from build123d import *

# Parameters (mm, degrees)
SKETCH1_W           = 101.6
SKETCH1_H           = 79
BOSS_EXTRUDE1_DEPTH = 3


with BuildPart() as part:
    # Sketch1 → Boss-Extrude1 (new body)
    with BuildSketch(Plane(origin=(0, 0, 0), x_dir=(1, 0, 0), z_dir=(0, 1, 0))):
        with Locations((44.42740929, 26.5)):
            Rectangle(SKETCH1_W, SKETCH1_H)
        with BuildLine():
            Line((9.87740929, 51.5), (9.87740929, 48.5))
            ThreePointArc((9.87740929, 48.5), (6.62740929, 45.25), (3.37740929, 48.5))
            Line((3.37740929, 48.5), (3.37740929, 51.5))
            ThreePointArc((3.37740929, 51.5), (6.62740929, 54.75), (9.87740929, 51.5))
        make_face(mode=Mode.SUBTRACT)
        with BuildLine():
            Line((9.87740929, 1.5), (9.87740929, -1.5))
            ThreePointArc((9.87740929, -1.5), (6.62740929, -4.75), (3.37740929, -1.5))
            Line((3.37740929, -1.5), (3.37740929, 1.5))
            ThreePointArc((3.37740929, 1.5), (6.62740929, 4.75), (9.87740929, 1.5))
        make_face(mode=Mode.SUBTRACT)
        with BuildLine():
            Line((59.87740929, 1.5), (59.87740929, -1.5))
            ThreePointArc((59.87740929, -1.5), (56.62740929, -4.75), (53.37740929, -1.5))
            Line((53.37740929, -1.5), (53.37740929, 1.5))
            ThreePointArc((53.37740929, 1.5), (56.62740929, 4.75), (59.87740929, 1.5))
        make_face(mode=Mode.SUBTRACT)
        with BuildLine():
            Line((85.47740929, 51.5), (85.47740929, 48.5))
            ThreePointArc((85.47740929, 48.5), (82.22740929, 45.25), (78.97740929, 48.5))
            Line((78.97740929, 48.5), (78.97740929, 51.5))
            ThreePointArc((78.97740929, 51.5), (82.22740929, 54.75), (85.47740929, 51.5))
        make_face(mode=Mode.SUBTRACT)
        with BuildLine():
            Line((78.97740929, 1.5), (78.97740929, -1.5))
            ThreePointArc((78.97740929, -1.5), (82.22740929, -4.75), (85.47740929, -1.5))
            Line((85.47740929, -1.5), (85.47740929, 1.5))
            ThreePointArc((85.47740929, 1.5), (82.22740929, 4.75), (78.97740929, 1.5))
        make_face(mode=Mode.SUBTRACT)
        with BuildLine():
            Line((28.97740929, 1.5), (28.97740929, -1.5))
            ThreePointArc((28.97740929, -1.5), (32.22740929, -4.75), (35.47740929, -1.5))
            Line((35.47740929, -1.5), (35.47740929, 1.5))
            ThreePointArc((35.47740929, 1.5), (32.22740929, 4.75), (28.97740929, 1.5))
        make_face(mode=Mode.SUBTRACT)
    extrude(amount=BOSS_EXTRUDE1_DEPTH)


solid = part.part
Model file for the job. Use its own axes, mm. A direction names the side the tool comes from. Coordinates: 2 decimals unless noted, no trailing zeros. Order: outer loops, then holes, each group sorted by start corner. A loop starts at its lowest first (then second) coordinate and runs counter-clockwise, first axis right, second up. Notation, with made-up numbers: (-1, 86.25) -> (5, 86.25) arc R19 cw to (5, 121.25) -> close; hole circle Ø3 at (89, 73). An arc over 180 degrees is marked (long way). Return JSON: item names as keys, results as strings. Group by question number.
Item 1: Saw through at C-C on x = 82.5. Write the cut outline in (y, z), then the cut area to 3 significant figures.
Item 2: Saw through at A-A on y = 1.35. Write the cut outline in (x, z).
Item 3: Wall check: line 1 along X through (y, z) = (0.35, -53); line 2 along Z through (x, y) = (55, 0.35); line 3 along Z through (x, y) = (7.5, 1.1). Give the ranges that are in metal, low to high. Write a range as [from, to].
Item 4: Saw through at D-D on z = -3. Write the cut outline in (x, y).
Item 5: Tool access for faces 4 (the flat face through (59.877, 1, 0)), 5 (the flat face through (95.227, 1, -26)): list every direction of +Z, -Z, +X, -X, +Y, -Y with a clear straight run to the whole face (end or side of a thin tool).
Item 6: Saw through at B-B on z = -46.5. Write the cut outline in (x, y), then the cut area to 3 significant figures.
Item 7: Pull direction Z, two halves, no side cores. Call faces 1 (the cylindrical face through (56.7, 1.48, 4.75)), 2 (the flat face through (44, 0, -27)), 3 (the flat face through (44, 1, -66)): pulls with the +Z half, pulls with the -Z half, needs draft (parallel to the pull), parting line crosses it, or undercut.
Values found:
{
 "1": {"outline": "(0, -66) -> (3, -66) -> (3, -54.74) -> (0, -54.74) -> close; (0, -45.26) -> (3, -45.26) -> (3, -4.74) -> (0, -4.74) -> close; (0, 4.74) -> (3, 4.74) -> (3, 13) -> (0, 13) -> close", "area": "180 mm2"},
 "2": {"outline": "(-6.37, -66) -> (95.23, -66) -> (95.23, 13) -> (-6.37, 13) -> close; hole (3.38, -51.5) arc R3.25 ccw to (9.88, -51.5) -> (9.88, -48.5) arc R3.25 ccw to (3.38, -48.5) -> close; hole (3.38, -1.5) arc R3.25 ccw to (9.88, -1.5) -> (9.88, 1.5) arc R3.25 ccw to (3.38, 1.5) -> close; hole (28.98, -1.5) arc R3.25 ccw to (35.48, -1.5) -> (35.48, 1.5) arc R3.25 ccw to (28.98, 1.5) -> close; hole (53.38, -1.5) arc R3.25 ccw to (59.88, -1.5) -> (59.88, 1.5) arc R3.25 ccw to (53.38, 1.5) -> close; hole (78.98, -51.5) arc R3.25 ccw to (85.48, -51.5) -> (85.48, -48.5) arc R3.25 ccw to (78.98, -48.5) -> close; hole (78.98, -1.5) arc R3.25 ccw to (85.48, -1.5) -> (85.48, 1.5) arc R3.25 ccw to (78.98, 1.5) -> close"},
 "3": {"line 1": "x = [-6.37, 3.74], [9.51, 79.34], [85.11, 95.23]", "line 2": "z = [-66, -4.31], [4.31, 13]", "line 3": "z = [-66, -54.63], [-45.37, -4.63], [4.63, 13]"},
 "4": {"outline": "(-6.37, 0) -> (3.74, 0) -> (3.74, 3) -> (-6.37, 3) -> close; (9.51, 0) -> (29.34, 0) -> (29.34, 3) -> (9.51, 3) -> close; (35.11, 0) -> (53.74, 0) -> (53.74, 3) -> (35.11, 3) -> close; (59.51, 0) -> (79.34, 0) -> (79.34, 3) -> (59.51, 3) -> close; (85.11, 0) -> (95.23, 0) -> (95.23, 3) -> (85.11, 3) -> close"},
 "5": {"face 4": "+Y, -Y", "face 5": "+Z, -Z, +X, +Y, -Y"},
 "6": {"outline": "(-6.37, 0) -> (4.07, 0) -> (4.07, 3) -> (-6.37, 3) -> close; (9.19, 0) -> (79.67, 0) -> (79.67, 3) -> (9.19, 3) -> close; (84.79, 0) -> (95.23, 0) -> (95.23, 3) -> (84.79, 3) -> close", "area": "274 mm2"},
 "7": {"face 1": "undercut", "face 2": "needs draft", "face 3": "pulls with the -Z half"}
}
